from build123d import *

# Parameters (mm, degrees)
CROQUIS1_R                               = 10
CROQUIS1_R_2                             = 1
SALIENTE_EXTRUIR1_DEPTH                  = 2
CROQUIS2_W                               = 8
CROQUIS2_H                               = 2
SALIENTE_EXTRUIR2_DEPTH                  = 5
TALADRO_DE_MARGEN_PARA_M1_61_D           = 1.7
TALADRO_DE_MARGEN_PARA_M1_61_CSINK_D     = 1.75
TALADRO_DE_MARGEN_PARA_M1_61_CSINK_ANGLE = 82


with BuildPart() as part:
    # Croquis1 → Saliente-Extruir1 (new body)
    with BuildSketch(Plane.XY):
        Circle(CROQUIS1_R)
        with Locations((-7.5, 0)):
            Circle(CROQUIS1_R_2, mode=Mode.SUBTRACT)
        with Locations((7.5, 0)):
            Circle(CROQUIS1_R_2, mode=Mode.SUBTRACT)
    extrude(amount=SALIENTE_EXTRUIR1_DEPTH)

    # Croquis2 → Saliente-Extruir2 (add)
    with BuildSketch(Plane.XY.offset(2)):
        with Locations((0, 2)):
            Rectangle(CROQUIS2_W, CROQUIS2_H)
        with Locations((0, -2)):
            Rectangle(CROQUIS2_W, CROQUIS2_H)
    extrude(amount=SALIENTE_EXTRUIR2_DEPTH)

    # Taladro de margen para M1.61 (through all)
    with Locations(Plane(origin=(0, -3, 0), x_dir=(-1, 0, 0), z_dir=(0, -1, 0))):
        with Locations((-2.65, -4.5), (2.65, -4.5)):
            CounterSinkHole(TALADRO_DE_MARGEN_PARA_M1_61_D / 2, TALADRO_DE_MARGEN_PARA_M1_61_CSINK_D / 2, counter_sink_angle=TALADRO_DE_MARGEN_PARA_M1_61_CSINK_ANGLE)


solid = part.part
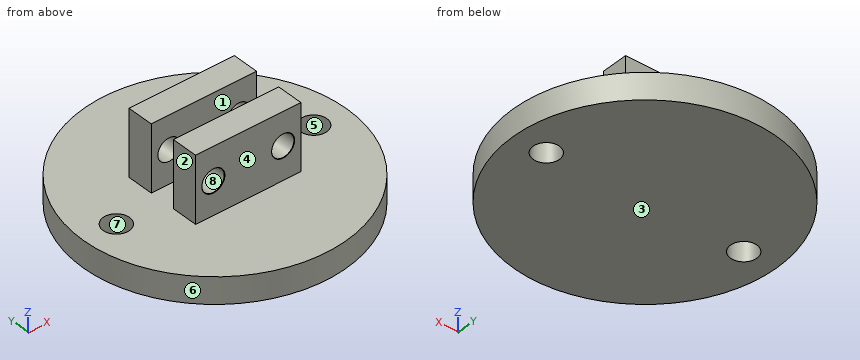
Here's how the part is built. I have some questions about the finished solid (model axes, mm). Face numbers are marked on the shaded views. A direction names the side the tool comes from. Round coordinates to 2 decimals unless told otherwise and drop trailing zeros. Loops run counter-clockwise (first coordinate to the right, second up) from the corner with the lowest first, then second, coordinate; pieces in that order, holes last. Notation, with made-up numbers: M 72.25,39.25 L 103.25,39.25 A17 ccw 103.25,56.25 Z; hole C -16.5,-20.75 d8. An arc over 180 degrees is marked long. Write each question's results on one line, items separated by ' | '. Start each with the question number.
(1) I want a section at B-B (x = 8). Please give me the cut outline in (y, z).
(2) I want a section at C-C (y = 2). Please give me the cut outline in (x, z), then the cut area to 3 significant figures.
(3) I want a section at A-A (z = 2.25). Please give me the cut outline in (x, y).
(4) Thinking about a two-plate mould opening in Y: for the marked faces 5, 6, 7 and 8, which applies, pulls with the +Y half, pulls with the -Y half, needs draft (parallel to the pull), parting line crosses it, or undercut?
(5) If I drill on probe 1 along X at (y, z) = (-2.55, 4.5); probe 2 along Z at (x, y) = (2.65, 1.9); probe 3 along Y at (x, z) = (2.25, 5.5), over which ranges is the centre line in solid material (lowest first)? Write a range as from..to.
(6) On a 3-axis mill with a long thin cutter (end or side, diameter ignored), from which of +Z, -Z, +X, -X, +Y, -Y can I reach the whole of each face in a straight line? I mean the marked faces 1, 2, 3 and 4. Say none if no direction works.
(7) I want a section at D-D (x = 2.65). Please give me the cut outline in (y, z) (3 decimals), then the cut area to 3 significant figures.
(8) Will these pins go through, and if not, where does the flat tip stop? P1, Ø1, axis at y = -1.5, z = 5.5, coming from the -X side; P2, Ø2.5, axis at x = 0.5, z = 4, coming from the +Y side; P3, Ø4, axis at x = -6.5, z = 5, coming from the +Y side; P4, Ø3, axis at y = 4.5, z = 3, coming from the -X side.
Solved:
1) outline: M -6,0 L -0.87,0 L -0.87,2 L -6,2 Z; M 0.87,0 L 6,0 L 6,2 L 0.87,2 Z
2) outline: M -9.8,0 L 9.8,0 L 9.8,2 L 4,2 L 4,7 L -4,7 L -4,2 L -9.8,2 Z; hole C -2.65,4.5 d1.7; hole C 2.65,4.5 d1.7 | area: 74.7 mm²
3) outline: M -4,-3 L 4,-3 L 4,-1 L -4,-1 Z; M -4,1 L 4,1 L 4,3 L -4,3 Z
4) face 5: undercut | face 6: parting line crosses it | face 7: undercut | face 8: needs draft
5) probe 1: x = -4..-3.5, -1.8..1.8, 3.5..4 | probe 2: z = 0..3.65, 5.35..7 | probe 3: y = -3..-1, 1..3
6) face 1: +Z, +X, -X | face 2: +Z, -X, +Y, -Y | face 3: -Z, +X, -X, +Y, -Y | face 4: +Z, +X, -X, -Y
7) outline: M -9.642,0 L 9.642,0 L 9.642,2 L 3,2 L 3,3.65 L 1,3.65 L 1,2 L -1,2 L -1,3.65 L -2.971,3.65 L -3,3.625 L -3,2 L -9.642,2 Z; M -3,5.375 L -2.971,5.35 L -1,5.35 L -1,7 L -3,7 Z; M 1,5.35 L 3,5.35 L 3,7 L 1,7 Z | area: 51.8 mm²
8) P1: stops at x = -4 | P2: stops at y = 3 | P3: passes through | P4: stops at x = -9.41
